Input: part model. Units: mm. Frame: model coordinates. Round coordinates to 2 decimals unless told otherwise and drop trailing zeros. Loops run counter-clockwise (first coordinate to the right, second up) from the corner with the lowest first, then second, coordinate; pieces in that order, holes last. Notation, with made-up numbers: M -21.75,59.25 L 25.25,59.25 A13 ccw 25.25,65.25 Z; hole C 23,44 d11. An arc over 180 degrees is marked long. Put each result on its own line as item: value. Start each with the question number.
1) Section B-B on z = 0.55. Output: boundary loops of the cut face in (x, y).
2) Section D-D on y = 24. Output: boundary loops of the cut face in (x, z).
3) Section C-C on x = -14. Output: boundary loops of the cut face in (y, z).
4) Line query: probe 1 along Y at (x, z) = (-4, 0.45); probe 2 along X at (y, z) = (51.5, 0.95); probe 3 along Y at (x, z) = (-12.5, 0.3). Output: solid intervals per line, ascending.
5) Section A-A on x = -5. Output: boundary loops of the cut face in (y, z).
Autodesk Inventor part; units mm, degrees
ref_plane "YZ Plane" through (0, 0, 0) normal (1, 0, 0) x (0, 1, 0)
ref_plane "XZ Plane" through (0, 0, 0) normal (0, 1, 0) x (-1, 0, 0)
ref_plane "XY Plane" through (0, 0, 0) normal (0, 0, 1) x (1, 0, 0)
sketch "Sketch2" plane through (0, 0, 0) normal (0, 0, 1) x (1, 0, 0)
  circle A0 centre (-4.7681, 50.6628) radius 2.39
  circle A1 centre (-4.7681, 50.6628) radius 2.39
  circle A2 centre (-5.08, 0) radius 2.1844
  circle A3 centre (-12.5662, 63.0568) radius 2.1844
  arc A4 (-10.1597, 0.0569) -> (0, 0) centre (-5.08, 0) ccw
  arc A5 (-8.1919, 65.6399) -> (-16.8387, 60.3087) centre (-12.5662, 63.0568) ccw
  line L0 (-16.8387, 60.3087) -> (-10.1261, 49.8724)
  line L1 (-0.6665, 52.8961) -> (-8.1919, 65.6399)
  line L2 (0, 0) -> (0, 50.4566)
  arc A6 (0, 50.4566) -> (-0.6665, 52.8961) centre (-4.7976, 50.4566) ccw
  line L3 (-9.6216, 48.1193) -> (-10.1597, 0.0569)
  arc A7 (-9.6216, 48.1193) -> (-10.1261, 49.8724) centre (-12.7964, 48.1549) ccw
  circle A8 centre (-12.5662, 63.0568) radius 2.1844
  circle A9 centre (-5.08, 0) radius 2.1844
  arc A10 (-10.1597, 0.0569) -> (0, 0) centre (-5.08, 0) ccw
  line L4 (-10.1597, 0.0569) -> (-9.6216, 48.1193)
  line L5 (-10.1261, 49.8724) -> (-16.8387, 60.3087)
  arc A11 (-9.6216, 48.1193) -> (-10.1261, 49.8724) centre (-12.7964, 48.1549) ccw
  arc A12 (-8.1919, 65.6399) -> (-16.8387, 60.3087) centre (-12.5662, 63.0568) ccw
  line L6 (-8.1919, 65.6399) -> (-0.6665, 52.8961)
extrude "Extrusion4" add sketch "Sketch2" along normal blind 1.62
properties part number "pneumaticwingplexi"
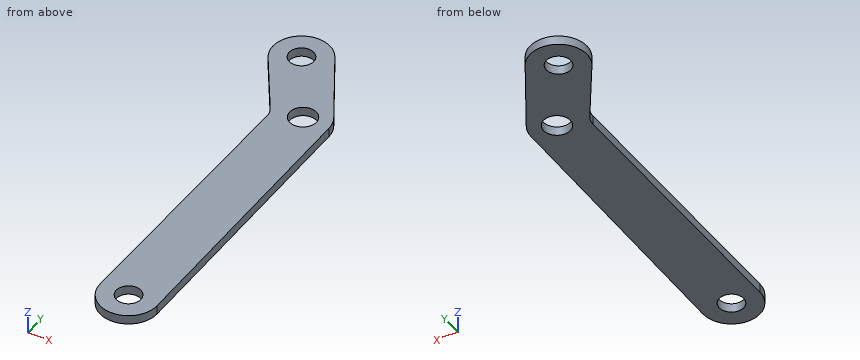
Geometry results:
1. outline: M -16.84,60.31 L -10.13,49.87 A3.17 cw -9.62,48.12 L -10.16,0.06 A5.08 ccw long 0,0 L 0,50.46 A4.8 ccw -0.67,52.9 L -8.19,65.64 A5.08 ccw long Z; hole C -12.57,63.06 d4.37; hole C -5.08,0 d4.37; hole C -4.77,50.66 d4.78
2. outline: M -9.89,0 L 0,0 L 0,1.62 L -9.89,1.62 Z
3. outline: M 55.9,0 L 61.41,0 L 61.41,1.62 L 55.9,1.62 Z; M 64.7,0 L 67.93,0 L 67.93,1.62 L 64.7,1.62 Z
4. probe 1: y = -4.96 to -1.9, 1.9 to 48.4, 52.93 to 58.54
4. probe 2: x = -11.17 to -7.01, -2.53 to -0.11
4. probe 3: y = 53.56 to 60.87, 65.24 to 68.14
5. outline: M -5.08,0 L -2.18,0 L -2.18,1.62 L -5.08,1.62 Z; M 2.18,0 L 48.28,0 L 48.28,1.62 L 2.18,1.62 Z; M 53.04,0 L 60.23,0 L 60.23,1.62 L 53.04,1.62 Z
